Here's how the part is built. I have some questions about the finished solid (model axes, mm). A direction names the side the tool comes from. Round coordinates to 2 decimals unless told otherwise and drop trailing zeros. Loops run counter-clockwise (first coordinate to the right, second up) from the corner with the lowest first, then second, coordinate; pieces in that order, holes last. Notation, with made-up numbers: (56.25, 77) -> (77.25, 77) arc R24 cw to (77.25, 106) -> close; hole circle Ø5 at (60.25, 65). An arc over 180 degrees is marked (long way). Use one line per item in the form item = value. Start each with the question number.
Item 1: If we section it at B-B (y = 12): State how many separate pieces and enclosed holes the cut face has, then the cut area to 3 significant figures.
Item 2: If we section it at A-A (x = -9): Write out the boundary of the cut face in (y, z).
Item 3: Thinking about a two-plate mould opening in X: for faces 1 (the face through (-15.5, -1, 8)), 2 (the face through (-5, -50, 5)), 3 (the face through (20, -1, 7)), which applies, released by +X, released by -X, zero draft, split by the parting line, or undercut?
Item 4: For faces 4 (the face through (11, -1, -3.9)), 5 (the face through (-15.21, -0.7, -4.15)), 6 (the face through (-11, -1, 3.9)), which set-ups out of +Z, -Z, +X, -X, +Y, -Y let a thin tool reach every point of the face, with its end or its side?
Item 5: I'm going to push flat-ended pins straight in: pin 1 Ø4 at (x, z) = (-14.5, 6) entering from -Y; pin 2 Ø3 at (y, z) = (-5.5, 1.5) entering from +X; pin 3 Ø1.4 at (x, y) = (12, 3.5) entering from +Z; pin 4 Ø2 at (x, y) = (12, -8.5) entering from -Z. Where does each tip first touch, or does it pass through?
Item 6: If I drill on L1, parallel to X at y = -3, z = -8; L2, parallel to Z at x = 10, y = 22.5; L3, parallel to Z at x = 14.5, y = 29.5, over which ranges is the centre line in solid material (lowest first)? Write a range as [from, to].
```python
from build123d import *

# Parameters (mm, degrees)
F1_DEPTH = 50
F2_R     = 1


with BuildPart() as f1:
    # F0 (on Front) → F1 (new body, symmetric)
    with BuildSketch(Plane.XZ):
        Polygon((-15.5, 6.5606601718), (-15.5, 8.4999998663), (-13.1, 8.4999998663), (-14.6, 9.9999998663), (-20, 9.9999998663), (-20, 4.5999998663), (-18.4999998663, 3.1), (-18.4999998663, 5.5), (-16.5606601718, 5.5), (-13.9, 2.8393398282), (-13.9, 0.1), (-13.7, 0.1), (-13.7, 0), (-13.7, -0.1), (-13.9, -0.1), (-13.9, -2.8393398282), (-16.5606601718, -5.5), (-18.4999998663, -5.5), (-18.4999998663, -3.1), (-20, -4.5999998663), (-20, -9.9999998663), (-14.6, -9.9999998663), (-13.1, -8.4999998663), (-15.5, -8.4999998663), (-15.5, -6.5606601718), (-12.8393398282, -3.9), (-10.1, -3.9), (-10.1, -3.7), (-9.9, -3.7), (-9.9, -3.9), (-7.1606601718, -3.9), (-4.5, -6.5606601718), (-4.5, -8.4999998663), (-6.9, -8.4999998663), (-5.4, -9.9999998663), (0, -9.9999998663), (5.4, -9.9999998663), (6.9, -8.4999998663), (4.5, -8.4999998663), (4.5, -6.5606601718), (7.1606601718, -3.9), (9.9, -3.9), (9.9, -3.7), (10.1, -3.7), (10.1, -3.9), (12.8393398282, -3.9), (15.5, -6.5606601718), (15.5, -8.4999998663), (13.1, -8.4999998663), (14.6, -9.9999998663), (20, -9.9999998663), (20, -4.5999998663), (18.4999998663, -3.1), (18.4999998663, -5.5), (16.5606601718, -5.5), (13.9, -2.8393398282), (13.9, -0.1), (13.7, -0.1), (13.7, 0), (13.7, 0.1), (13.9, 0.1), (13.9, 2.8393398282), (16.5606601718, 5.5), (18.4999998663, 5.5), (18.4999998663, 3.1), (20, 4.5999998663), (20, 9.9999998663), (14.6, 9.9999998663), (13.1, 8.4999998663), (15.5, 8.4999998663), (15.5, 6.5606601718), (12.8393398282, 3.9), (10.1, 3.9), (10.1, 3.7), (9.9, 3.7), (9.9, 3.9), (7.1606601718, 3.9), (4.5, 6.5606601718), (4.5, 8.4999998663), (6.9, 8.4999998663), (5.4, 9.9999998663), (0, 9.9999998663), (-5.4, 9.9999998663), (-6.9, 8.4999998663), (-4.5, 8.4999998663), (-4.5, 6.5606601718), (-7.1606601718, 3.9), (-9.9, 3.9), (-9.9, 3.7), (-10.1, 3.7), (-10.1, 3.9), (-12.8393398282, 3.9), align=None)
        with BuildLine():
            ThreePointArc((-12.1, 0), (-10, 2.1), (-7.9, 0))
            ThreePointArc((-7.9, 0), (-10, -2.1), (-12.1, 0))
        make_face(mode=Mode.SUBTRACT)
        Polygon((-6.1, 2.8393398282), (-2.8, 6.1393398282), (-2.8, 8.4999998663), (0, 8.4999998663), (2.8, 8.4999998663), (2.8, 6.1393398282), (6.1, 2.8393398282), (6.1, 0), (6.1, -2.8393398282), (2.8, -6.1393398282), (2.8, -8.4999998663), (0, -8.4999998663), (-2.8, -8.4999998663), (-2.8, -6.1393398282), (-6.1, -2.8393398282), (-6.1, 0), align=None, mode=Mode.SUBTRACT)
        with BuildLine():
            ThreePointArc((12.1, 0), (10, -2.1), (7.9, 0))
            ThreePointArc((7.9, 0), (10, 2.1), (12.1, 0))
        make_face(mode=Mode.SUBTRACT)
    extrude(amount=F1_DEPTH, both=True)

    # F2
    f2_edges = [f1.edges().sort_by_distance(p)[0] for p in [
        (-20, 0, 10),
        (20, 0, 10),
        (20, 0, -10),
        (-20, 0, -10),
    ]]
    fillet(f2_edges, radius=F2_R)


solid = f1.part
```
Values found:
q1.separate_pieces = 1
q1.enclosed_holes = 3
q1.area = 286 mm2
q2.outline = (-50, -3.9) -> (50, -3.9) -> (50, -1.85) -> (-50, -1.85) -> close; (-50, 1.85) -> (50, 1.85) -> (50, 3.9) -> (-50, 3.9) -> close
q3.face_1 = undercut
q3.face_2 = zero draft
q3.face_3 = released by +X
q4.face_4 = -Z, +Y, -Y
q4.face_5 = +Y, -Y
q4.face_6 = +Z, +Y, -Y
q5.pin_1 = -50
q5.pin_2 = 14.06
q5.pin_3 = 3.9
q5.pin_4 = -4.06
q6.L1 = [-20, -15.5], [-4.5, -2.8], [2.8, 4.5], [15.5, 20]
q6.L2 = [-3.7, -2.1], [2.1, 3.7]
q6.L3 = [-9.9, -8.5], [-5.56, -3.44], [3.44, 5.56], [8.5, 9.9]
